Source: CAD feature listing. Evaluate the final solid. Frame: model axes, mm. A direction names the side the tool comes from. Give positions to 0.01 mm unless a question says otherwise; leave off trailing zeros. Loops run counter-clockwise (first coordinate to the right, second up) from the corner with the lowest first, then second, coordinate; pieces in that order, holes last. Notation, with made-up numbers: M -13,50 L 13,50 A30 ccw 13,78 Z; hole C -16.5,35 d5. An arc over 180 degrees is marked long. Answer in a Markdown table with one row per item.
```python
from build123d import *

# Parameters (mm, degrees)
F0_W     = 8.636
F0_H     = 25.4
F1_DEPTH = 6.35
F2_W     = 8.636
F2_H     = 4.064
F3_DEPTH = 10.16
F4_R     = 1.190625
F5_DEPTH = 16.511
F7_R     = 2.099945
F8_DEPTH = 5.08


with BuildPart() as f1:
    # F0 (on Right) → F1 (new body)
    with BuildSketch(Plane.YZ):
        with Locations((4.318, 12.7)):
            Rectangle(F0_W, F0_H)
    extrude(amount=F1_DEPTH)

    # F2 (on face) → F3 (join)
    with BuildSketch(Plane.YZ.offset(6.35)):
        with Locations((4.318, 23.368)):
            Rectangle(F2_W, F2_H)
    extrude(amount=F3_DEPTH)

    # F4 (on face) → F5 (cut, through all)
    with BuildSketch(Plane.YZ.offset(16.51)):
        with Locations((4.318, 23.368)):
            Circle(F4_R)
    extrude(amount=-F5_DEPTH, mode=Mode.SUBTRACT)

    # F7 (on face) → F8 (cut)
    with BuildSketch(Plane(origin=(0, 0, 0), x_dir=(0, -1, 0), z_dir=(-1, 0, 0))):
        with Locations((-4.315846, 22.864808)):
            Circle(F7_R)
    extrude(amount=-F8_DEPTH, mode=Mode.SUBTRACT)


solid = f1.part
```
Q1. Mould query, pull axis Y, two halves, no side actions, for faces 4 (the flat face through (11, 4, 21.336)), 5 (the flat face through (4, 8.636, 13)), 6 (the cylindrical face through (10.875, 4.06, 22.206)). Classes: +Y half, -Y half, draft (parallel to the pull), parting line (faces both ways), or undercut.
Values follow:
| item | result |
|---|---|
| face 4 | draft |
| face 5 | +Y half |
| face 6 | undercut |
Q2. Section query C-C (x = 13.75). Output: boundary loops of the cut face in (y, z).
Values follow:
| item | result |
|---|---|
| outline | M 0,21.34 L 8.64,21.34 L 8.64,25.4 L 0,25.4 Z; hole C 4.32,23.37 d2.38 |
Q3. Reachability of faces 1 (the flat face through (3, 4, 0)), 2 (the cylindrical face through (2.504, 5.982, 21.587)), 3 (the flat face through (6.35, 4, 11)) from +Z, -Z, +X, -X, +Y, -Y: full face, straight path, thin tool, end or side. Return the list, or none.
Values follow:
| item | result |
|---|---|
| face 1 | -Z, +X, -X, +Y, -Y |
| face 2 | -X |
| face 3 | -Z, +X, +Y, -Y |
Q4. Section query A-A (z = 22.5). Output: boundary loops of the cut face in (x, y), plus the area to 3 significant figures.
Values follow:
| item | result |
|---|---|
| outline | M 0,0 L 16.51,0 L 16.51,3.5 L 5.08,3.5 L 5.08,2.25 L 0,2.25 Z; M 0,6.38 L 5.08,6.38 L 5.08,5.13 L 16.51,5.13 L 16.51,8.64 L 0,8.64 Z |
| area | 103 mm^2 |
Q5. Ray query, probe 1 along Z at (x, y) = (6.5, 7.25); probe 2 along X at (y, z) = (2.5, 18.75); probe 3 along X at (y, z) = (3, 23.5). Return the intervals inside material, ascending. Write a range as from..to.
Values follow:
| item | result |
|---|---|
| probe 1 | 21.34..25.4 |
| probe 2 | 0..6.35 |
| probe 3 | 5.08..16.51 |
Q6. Contact query for flat-ended pins moving along their axis: pin 1 Ø4 at (y, z) = (4.318, 23.368) entering from -X; pin 2 Ø1.5 at (x, y) = (13, 7) entering from -Z; pin 3 Ø1 at (y, z) = (6, 5) entering from +X; pin 4 Ø1.3 at (y, z) = (5, 23.5) entering from -X. Output: stop coordinate, or through.
Values follow:
| item | result |
|---|---|
| pin 1 | x = 0 |
| pin 2 | z = 21.34 |
| pin 3 | x = 6.35 |
| pin 4 | x = 5.08 |
Q7. Section query B-B (y = 1.75). Output: boundary loops of the cut face in (x, z), plus the area to 3 significant figures.
Values follow:
| item | result |
|---|---|
| outline | M 0,0 L 6.35,0 L 6.35,21.34 L 16.51,21.34 L 16.51,25.4 L 0,25.4 Z |
| area | 203 mm^2 |
Q8. Section query D-D (z = 6). Output: boundary loops of the cut face in (x, y).
Values follow:
| item | result |
|---|---|
| outline | M 0,0 L 6.35,0 L 6.35,8.64 L 0,8.64 Z |
